from build123d import *

# Parameters (mm, degrees)
F0_W     = 300
F0_H     = 300
F1_DEPTH = 300
F2_T     = -12
F3_W     = 276
F3_H     = 12
F4_DEPTH = 295


with BuildPart() as f1:
    # F0 (on Front) → F1 (new body)
    with BuildSketch(Plane.XZ):
        Rectangle(F0_W, F0_H)
    extrude(amount=-F1_DEPTH)

    # F2
    f2_openings = [f1.faces().sort_by_distance(p)[0] for p in [
        (0, 0, 0),
    ]]
    offset(amount=F2_T, openings=f2_openings)

    # F3 (on face) → F4 (join)
    with BuildSketch(Plane.XZ):
        Rectangle(F3_W, F3_H)
    extrude(amount=-F4_DEPTH)


solid = f1.part
CAD build for the part. Positions are in the model's coordinates, mm. A direction names the side the tool comes from. Give positions to 0.01 mm unless a question says otherwise; leave off trailing zeros. Order: outer loops, then holes, each group sorted by start corner. A loop starts at its lowest first (then second) coordinate and runs counter-clockwise, first axis right, second up. Notation, with made-up numbers: (39.5, -36) -> (82.5, -36) arc R23 ccw to (82.5, -5) -> close; hole circle Ø11 at (23, 27). An arc over 180 degrees is marked (long way). Return JSON: item names as keys, results as strings.
Q1. Which spindle directions (+Z, -Z, +X, -X, +Y, -Y) get a long thin tool onto all of the face, cutting with end or side? Do faces 1 (the face through (-2, 288, 73)), 2 (the face through (-2, 300, 2)). Say none if no direction does.
Working result:
{"face 1": "-Y", "face 2": "+Z, -Z, +X, -X, +Y"}
Q2. Saw through at B-B (y = 136.5). Write the cut outline in (x, z), then the cut area to 3 significant figures.
Working result:
{"outline": "(-150, -150) -> (150, -150) -> (150, 150) -> (-150, 150) -> close; hole (-138, -138) -> (138, -138) -> (138, -6) -> (-138, -6) -> close; hole (-138, 6) -> (138, 6) -> (138, 138) -> (-138, 138) -> close", "area": "17,100 mm²"}
Q3. Drill centre lines: line 1 (Z direction, x = 84, y = 18); line 2 (X direction, y = 28, z = -101.5); line 3 (Y direction, x = 74, z = 65.5). Where is each one in solid material? Low to high.
Working result:
{"line 1": "-150 to -138, -6 to 6, 138 to 150", "line 2": "-150 to -138, 138 to 150", "line 3": "288 to 300"}
Q4. Mould opens along X. For faces 3 (the face through (-1, 0, 1)), 4 (the face through (-2, 142, 138)), 5 (the face through (150, 148, -2)) say: pulls with the +X half, pulls with the -X half, needs draft (parallel to the pull), parting line crosses it, or undercut.
Working result:
{"face 3": "needs draft", "face 4": "undercut", "face 5": "pulls with the +X half"}
Q5. Flat gauge pin, fed straight in: pin 1 (4 mm diameter, centred on x = -107.5, z = 37.5, fed in from -Y). Where does the tip first touch, or does it go through?
Working result:
{"pin 1": "y = 288"}
Q6. Saw through at C-C (x = 121.5). Write the cut outline in (y, z).
Working result:
{"outline": "(0, -150) -> (300, -150) -> (300, 150) -> (0, 150) -> (0, 138) -> (288, 138) -> (288, 6) -> (0, 6) -> (0, -6) -> (288, -6) -> (288, -138) -> (0, -138) -> close"}
Q7. Saw through at A-A (z = -15.5). Write the cut outline in (x, y), then the cut area to 3 significant figures.
Working result:
{"outline": "(-150, 0) -> (-138, 0) -> (-138, 288) -> (138, 288) -> (138, 0) -> (150, 0) -> (150, 300) -> (-150, 300) -> close", "area": "10,500 mm²"}
